Geometry check sheet. Reference: the model listing, model coordinates, mm. Face numbers are marked on the shaded views. A direction names the side the tool comes from. Give positions to 0.01 mm unless a question says otherwise; leave off trailing zeros. Loops run counter-clockwise (first coordinate to the right, second up) from the corner with the lowest first, then second, coordinate; pieces in that order, holes last.
1. Release check for a two-part mould opening along Z. For the marked faces 4, 5 and 6 record: +Z half, -Z half, draft (parallel to the pull), parting line (faces both ways), or undercut.
2. Cross-section at C-C, the plane z = 1440. Record the cut outline in (x, y).
3. Cross-section at A-A, the plane y = -200. Record the cut outline in (x, z), plus the area to 3 significant figures.
4. Cross-section at B-B, the plane x = 498. Record the cut outline in (y, z), plus the area to 3 significant figures.
5. Material ranges on L1, parallel to X at y = -312, z = 1629; L2, parallel to Z at x = 752, y = -602.5; L3, parallel to Y at x = 482, z = 2060.5, recorded low to high.
6. Go/stop test with flat-tipped pins: pin 1 Ø8 at (x, y) = (179.5, -196) entering from -Z; pin 2 Ø8 at (x, z) = (816, 612.5) entering from -Y. Record where each tip stops, or that it passes through.
7. Tool access check on the marked faces 1, 2 and 3. Record the directions out of +Z, -Z, +X, -X, +Y, -Y that give a thin tool (end or side, any length) a straight path to the whole face; none if there is none.
from build123d import *

# Parameters (mm, degrees)
F0_W     = 711.2
F0_H     = 2324.1
F1_DEPTH = 914.4
F2_W     = 838.2
F2_H     = 1828.8
F2_H_2   = 400.05
F3_DEPTH = 698.5


with BuildPart() as f1:
    # F0 (on Right) → F1 (new body)
    with BuildSketch(Plane.YZ):
        with Locations((-355.6, 1162.05)):
            Rectangle(F0_W, F0_H)
    extrude(amount=F1_DEPTH)

    # F2 (on face) → F3 (cut)
    with BuildSketch(Plane.XZ.offset(711.2)):
        with Locations((457.2, 914.4)):
            Rectangle(F2_W, F2_H)
        with Locations((457.2, 2066.925)):
            Rectangle(F2_W, F2_H_2)
    extrude(amount=-F3_DEPTH, mode=Mode.SUBTRACT)


solid = f1.part
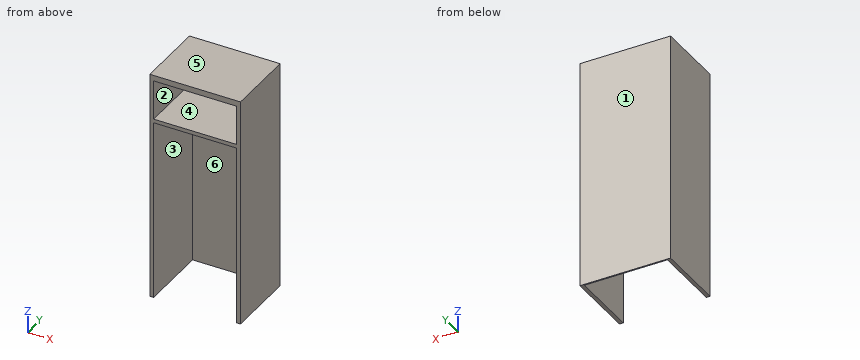
Result:
1. face 4: undercut
1. face 5: +Z half
1. face 6: draft
2. outline: (0, -711.2) - (38.1, -711.2) - (38.1, -12.7) - (876.3, -12.7) - (876.3, -711.2) - (914.4, -711.2) - (914.4, 0) - (0, 0) - close
3. outline: (0, 0) - (38.1, 0) - (38.1, 1828.8) - (876.3, 1828.8) - (876.3, 0) - (914.4, 0) - (914.4, 2324.1) - (0, 2324.1) - close; hole (38.1, 1866.9) - (876.3, 1866.9) - (876.3, 2266.95) - (38.1, 2266.95) - close
3. area: 257,000 mm2
4. outline: (-711.2, 1828.8) - (-12.7, 1828.8) - (-12.7, 0) - (0, 0) - (0, 2324.1) - (-711.2, 2324.1) - (-711.2, 2266.95) - (-12.7, 2266.95) - (-12.7, 1866.9) - (-711.2, 1866.9) - close
4. area: 96,000 mm2
5. L1: x = 0 to 38.1, 876.3 to 914.4
5. L2: z = 1828.8 to 1866.9, 2266.95 to 2324.1
5. L3: y = -12.7 to 0
6. pin 1: stops at z = 1828.8
6. pin 2: stops at y = -12.7
7. face 1: +Z, -Z, +X, -X, +Y
7. face 2: -Y
7. face 3: -Z, -Y
